Design review of the part shown in the three views and the two pictorial views. Dimensions are in mm from the part's minimum x, y and z. Give positions to 0.01 mm unless a question says otherwise; leave off trailing zeros. Loops run counter-clockwise (first coordinate to the right, second up) from the corner with the lowest first, then second, coordinate; pieces in that order, holes last.
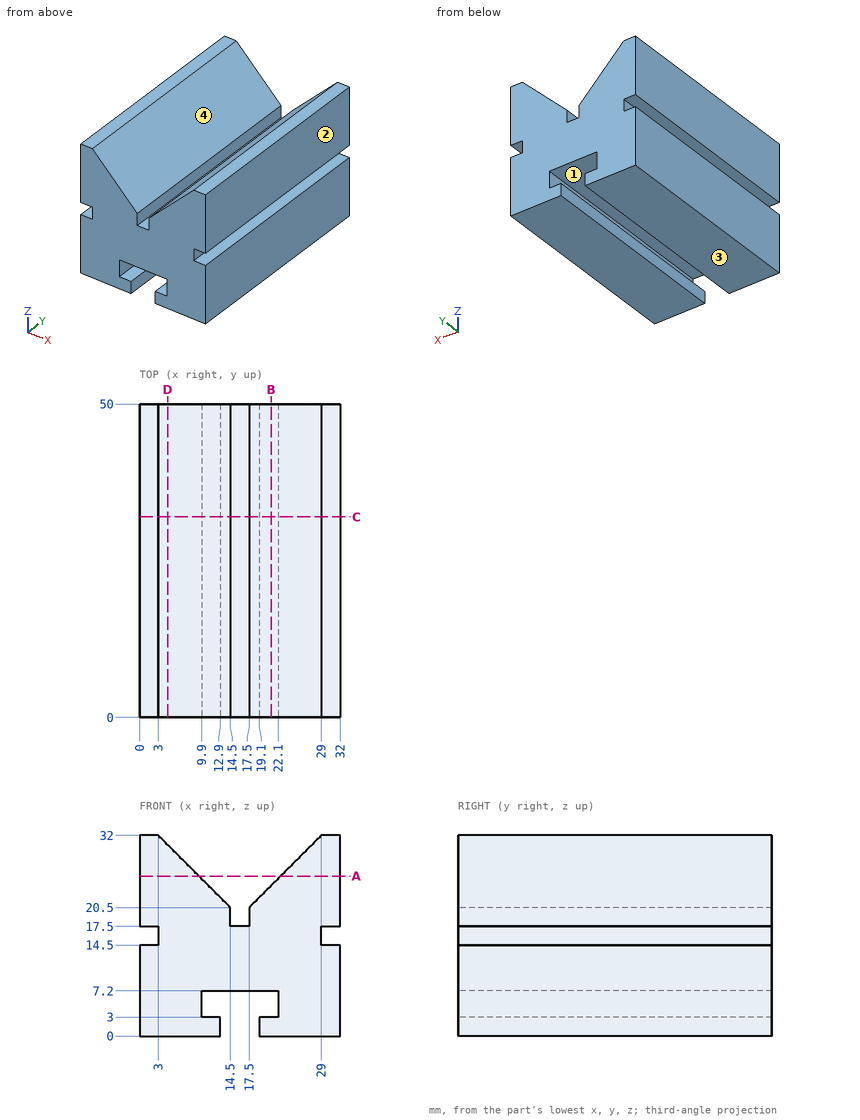
Q1. For probe 1 along X at (y, z) = (17, 4.5); probe 2 along X at (y, z) = (46.5, 19.5), list the stretches that pass through material, from the lowest coordinate up.
Answers:
probe 1: x = 0 to 9.9, 22.1 to 32
probe 2: x = 0 to 14.5, 17.5 to 32
Q2. Mouldability with a two-part tool opening along Z and no side actions: class the marked faces 1, 2, 3 and 4 as +Z half, -Z half, draft (parallel to the pull), parting line (faces both ways), or undercut.
Answers:
face 1: undercut
face 2: draft
face 3: -Z half
face 4: +Z half
Q3. Consider section C-C on y = 32. Give the boundary of the cut face in (x, z).
Answers:
outline: (0, 0) - (12.9, 0) - (12.9, 3) - (9.9, 3) - (9.9, 7.2) - (22.1, 7.2) - (22.1, 3) - (19.1, 3) - (19.1, 0) - (32, 0) - (32, 14.5) - (29, 14.5) - (29, 17.5) - (32, 17.5) - (32, 32) - (29, 32) - (17.5, 20.5) - (17.5, 17.5) - (14.5, 17.5) - (14.5, 20.5) - (3, 32) - (0, 32) - (0, 17.5) - (3, 17.5) - (3, 14.5) - (0, 14.5) - close
Q4. Consider section B-B on x = 21. Give the boundary of the cut face in (y, z), plus the area to 3 significant figures.
Answers:
outline: (0, 0) - (50, 0) - (50, 3) - (0, 3) - close; (0, 7.2) - (50, 7.2) - (50, 24) - (0, 24) - close
area: 990 mm2
Q5. For pin 1 Ø2.5 at (x, y) = (11.5, 33.5) entering from +Z; pin 2 Ø0.9 at (x, y) = (15.5, 29) entering from +Z, all flat-tipped, find the tip position at first contact; note any pin that passes through.
Answers:
pin 1: stops at z = 24.75
pin 2: stops at z = 17.5
Q6. Consider section D-D on x = 4.5. Give the boundary of the cut face in (y, z).
Answers:
outline: (0, 0) - (50, 0) - (50, 30.5) - (0, 30.5) - close
Q7. Consider section A-A on z = 25.5. Give the boundary of the cut face in (x, y).
Answers:
outline: (0, 0) - (9.5, 0) - (9.5, 50) - (0, 50) - close; (22.5, 0) - (32, 0) - (32, 50) - (22.5, 50) - close
